```python
from build123d import *

# Parameters (mm, degrees)
SKETCH091_R          = 3
PAD031_DEPTH         = 10
SKETCH092_R          = 2.5
POCKET026_DEPTH      = 15.001
POCKET026_DEPTH_BACK = -15.001


with BuildPart() as part:
    # Sketch091 → Pad031 (new body)
    with BuildSketch(Plane.XZ):
        with BuildLine():
            Line((-2.65, 15), (9.65, 15))
            ThreePointArc((16, 8.65), (14.140128, 13.140128), (9.65, 15))
            Line((16, 8.65), (16, -8.65))
            ThreePointArc((9.65, -15), (14.140128, -13.140128), (16, -8.65))
            Line((9.65, -15), (-2.65, -15))
            ThreePointArc((-9, -8.65), (-7.140128, -13.140128), (-2.65, -15))
            Line((-9, -8.65), (-9, -6))
            Line((5, -6), (-9, -6))
            ThreePointArc((5, -6), (7.12132, -5.12132), (8, -3))
            Line((8, 3), (8, -3))
            ThreePointArc((8, 3), (7.12132, 5.12132), (5, 6))
            Line((-9, 6), (5, 6))
            Line((-9, 6), (-9, 8.65))
            ThreePointArc((-2.65, 15), (-7.140128, 13.140128), (-9, 8.65))
        make_face()
        with Locations((10, 10)):
            Circle(SKETCH091_R, mode=Mode.SUBTRACT)
        with BuildLine():
            ThreePointArc((13, -9.5), (10, -6.5), (7, -9.5))
            Line((7, -9.5), (7, -10.5))
            ThreePointArc((7, -10.5), (10, -13.5), (13, -10.5))
            Line((13, -9.5), (13, -10.5))
        make_face(mode=Mode.SUBTRACT)
    extrude(amount=PAD031_DEPTH)

    # Sketch092 → Pocket026 (cut, two sides)
    with BuildSketch(Plane.XY) as pocket026_sk:
        with Locations((-1, -5)):
            Circle(SKETCH092_R)
    extrude(amount=-POCKET026_DEPTH, mode=Mode.SUBTRACT)
    extrude(pocket026_sk.sketch, amount=-POCKET026_DEPTH_BACK, mode=Mode.SUBTRACT)


solid = part.part
```
Read the model definition and answer for the solid it produces. Units are mm, in the model's axes. A direction names the side the tool comes from. Coordinates: 2 decimals unless noted, no trailing zeros. Loops run counter-clockwise (first coordinate to the right, second up) from the corner with the lowest first, then second, coordinate; pieces in that order, holes last. Notation, with made-up numbers: (5, 86.5) -> (32, 86.5) arc R25 ccw to (32, 115.5) -> close; hole circle Ø1 at (26.25, -10). An arc over 180 degrees is marked (long way). Return JSON: item names as keys, results as strings.
Item 1: Find section C-C (y = -8). Determine the outline of the cut face in (x, z).
Answers:
{"outline": "(-9, -8.65) arc R6.35 ccw to (-2.65, -15) -> (9.65, -15) arc R6.35 ccw to (16, -8.65) -> (16, 8.65) arc R6.35 ccw to (9.65, 15) -> (-2.65, 15) arc R6.35 ccw to (-9, 8.65) -> (-9, 6) -> (5, 6) arc R3 cw to (8, 3) -> (8, -3) arc R3 cw to (5, -6) -> (-9, -6) -> close; hole (7, -10.5) arc R3 ccw to (13, -10.5) -> (13, -9.5) arc R3 ccw to (7, -9.5) -> close; hole circle Ø6 at (10, 10)"}
Item 2: For a pull along X with two mould halves and no side action, classify faces 1 (the flat face through (13, -5, -10)), 2 (the flat face through (9, -10, 0)), 3 (the cylindrical face through (-7.09, -4.93, 13.19)) as +X half, -X half, draft (parallel to the pull), parting line (faces both ways), or undercut.
Answers:
{"face 1": "undercut", "face 2": "draft", "face 3": "-X half"}
Item 3: Find section A-A (z = 10). Determine the outline of the cut face in (x, y), plus the area to 3 significant figures.
Answers:
{"outline": "(-8.85, -10) -> (7, -10) -> (7, 0) -> (-8.85, 0) -> close; (13, -10) -> (15.85, -10) -> (15.85, 0) -> (13, 0) -> close; hole circle Ø5 at (-1, -5)", "area": "167 mm2"}
Item 4: Flat-ended cylindrical pins translate along their axes: P1, Ø1.1, axis at y = -6.5, z = -10, coming from the +X side; P2, Ø1.5, axis at y = -3, z = 1, coming from the -X side; P3, Ø2, axis at x = 12, y = -2, coming from the -Z side; P4, Ø4.5, axis at x = -1, y = -5, coming from the -Z side. Find the tip coordinate at first contact, or state that the pin passes through.
Answers:
{"P1": "stops at x = 15.95", "P2": "stops at x = 8", "P3": "stops at z = -14.85", "P4": "passes through"}
Item 5: Find section B-B (x = 4.5). Determine the outline of the cut face in (y, z), plus the area to 3 significant figures.
Answers:
{"outline": "(-10, -15) -> (0, -15) -> (0, -6) -> (-10, -6) -> close; (-10, 6) -> (0, 6) -> (0, 15) -> (-10, 15) -> close", "area": "180 mm2"}
Item 6: Find the intervals of material crossed by probe 1 along Y at (x, z) = (-1, -10.75); probe 2 along X at (y, z) = (-5, 11.25); probe 3 along X at (y, z) = (-5, 8.5), in increasing order.
Answers:
{"probe 1": "y = -10 to -7.5, -2.5 to 0", "probe 2": "x = -8.44 to -3.5, 1.5 to 7.27, 12.73 to 15.44", "probe 3": "x = -9 to -3.5, 1.5 to 7.4, 12.6 to 16"}
Item 7: For faces 4 (the flat face through (-9, -5, 7)), 5 (the flat face through (7, -5, -10)), 6 (the flat face through (-4, -5, 6)), determine the directions among +Z, -Z, +X, -X, +Y, -Y from which every point of the face is accessible in a straight line to the end or side of a thin tool.
Answers:
{"face 4": "+Z, -Z, -X, +Y, -Y", "face 5": "+Y, -Y", "face 6": "-X, +Y, -Y"}
Item 8: Find section D-D (y = -5). Determine the outline of the cut face in (x, z), plus the area to 3 significant figures.
Answers:
{"outline": "(-9, -8.65) arc R6.35 ccw to (-3.5, -14.94) -> (-3.5, -6) -> (-9, -6) -> close; (-9, 6) -> (-3.5, 6) -> (-3.5, 14.94) arc R6.35 ccw to (-9, 8.65) -> close; (1.5, -15) -> (9.65, -15) arc R6.35 ccw to (16, -8.65) -> (16, 8.65) arc R6.35 ccw to (9.65, 15) -> (1.5, 15) -> (1.5, 6) -> (5, 6) arc R3 cw to (8, 3) -> (8, -3) arc R3 cw to (5, -6) -> (1.5, -6) -> close; hole (7, -10.5) arc R3 ccw to (13, -10.5) -> (13, -9.5) arc R3 ccw to (7, -9.5) -> close; hole circle Ø6 at (10, 10)", "area": "363 mm2"}
